Model file for the job. Use its own axes, mm. Round coordinates to 2 decimals unless told otherwise and drop trailing zeros. Use one line per item in the form item = value.
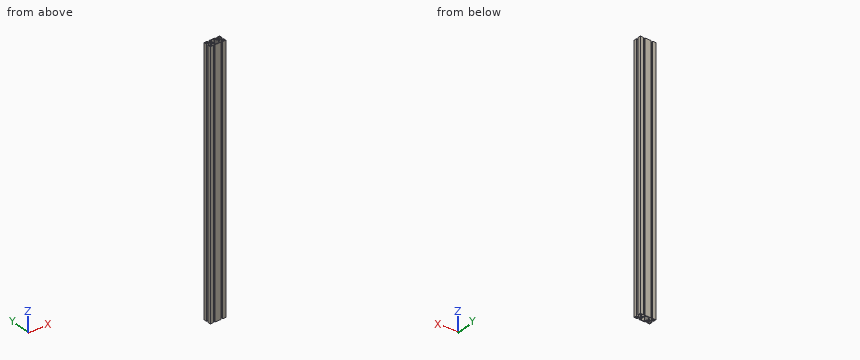
from build123d import *

# Parameters (mm, degrees)
F0_R     = 3
F0_R_2   = 2.5
F1_DEPTH = 1000
F2_R     = 2
F3_R     = 7


# Not quite as in the source:
# - a feature names something its author has since deleted; it is built from what else it names


with BuildPart() as f1:
    # F0 (on Top) → F1 (new body)
    with BuildSketch(Plane.XY):
        with BuildLine():
            Line((18.15, -15), (30, -15))
            Line((30, -15), (30, -3.15))
            Line((30, -3.15), (27.5, -3.15))
            Line((27.5, -3.15), (27.5, -5.15))
            Line((27.5, -5.15), (21.5477069044, -5.15))
            ThreePointArc((21.5477069044, -5.15), (19.5, 0), (21.5477069044, 5.15))
            Line((21.5477069044, 5.15), (27.5, 5.15))
            Line((27.5, 5.15), (27.5, 3.15))
            Line((27.5, 3.15), (30, 3.15))
            Line((30, 3.15), (30, 15))
            Line((30, 15), (18.15, 15))
            Line((18.15, 15), (18.15, 12.5))
            Line((18.15, 12.5), (20.15, 12.5))
            Line((20.15, 12.5), (20.15, 6.5477069044))
            ThreePointArc((20.15, 6.5477069044), (15, 4.5), (9.85, 6.5477069044))
            Line((9.85, 6.5477069044), (9.85, 12.5))
            Line((9.85, 12.5), (11.85, 12.5))
            Line((11.85, 12.5), (11.85, 15))
            Line((11.85, 15), (-11.85, 15))
            Line((-11.85, 15), (-11.85, 12.5))
            Line((-11.85, 12.5), (-9.85, 12.5))
            Line((-9.85, 12.5), (-9.85, 6.5477069044))
            ThreePointArc((-9.85, 6.5477069044), (-15, 4.5), (-20.15, 6.5477069044))
            Line((-20.15, 6.5477069044), (-20.15, 12.5))
            Line((-20.15, 12.5), (-18.15, 12.5))
            Line((-18.15, 12.5), (-18.15, 15))
            Line((-18.15, 15), (-30, 15))
            Line((-30, 15), (-30, 3.15))
            Line((-30, 3.15), (-27.5, 3.15))
            Line((-27.5, 3.15), (-27.5, 5.15))
            Line((-27.5, 5.15), (-21.5477069044, 5.15))
            ThreePointArc((-21.5477069044, 5.15), (-19.5, 0), (-21.5477069044, -5.15))
            Line((-21.5477069044, -5.15), (-27.5, -5.15))
            Line((-27.5, -5.15), (-27.5, -3.15))
            Line((-27.5, -3.15), (-30, -3.15))
            Line((-30, -3.15), (-30, -15))
            Line((-30, -15), (-18.15, -15))
            Line((-18.15, -15), (-18.15, -12.5))
            Line((-18.15, -12.5), (-20.15, -12.5))
            Line((-20.15, -12.5), (-20.15, -6.5477069044))
            ThreePointArc((-20.15, -6.5477069044), (-15, -4.5), (-9.85, -6.5477069044))
            Line((-9.85, -6.5477069044), (-9.85, -12.5))
            Line((-9.85, -12.5), (-11.85, -12.5))
            Line((-11.85, -12.5), (-11.85, -15))
            Line((-11.85, -15), (11.85, -15))
            Line((11.85, -15), (11.85, -12.5))
            Line((11.85, -12.5), (9.85, -12.5))
            Line((9.85, -12.5), (9.85, -6.5477069044))
            ThreePointArc((9.85, -6.5477069044), (15, -4.5), (20.15, -6.5477069044))
            Line((20.15, -6.5477069044), (20.15, -12.5))
            Line((20.15, -12.5), (18.15, -12.5))
            Line((18.15, -12.5), (18.15, -15))
        make_face()
        with Locations((-25, -10)):
            Circle(F0_R, mode=Mode.SUBTRACT)
        with Locations((25, -10)):
            Circle(F0_R, mode=Mode.SUBTRACT)
        with Locations((-15, 0)):
            Circle(F0_R_2, mode=Mode.SUBTRACT)
        with Locations((-25, 10)):
            Circle(F0_R, mode=Mode.SUBTRACT)
        Polygon((-7, 7), (-7, 12.5), (0, 12.5), (7, 12.5), (7, 7), (10, 0), (7, -7), (7, -12.5), (0, -12.5), (-7, -12.5), (-7, -7), (-10, 0), align=None, mode=Mode.SUBTRACT)
        with Locations((15, 0)):
            Circle(F0_R_2, mode=Mode.SUBTRACT)
        with Locations((25, 10)):
            Circle(F0_R, mode=Mode.SUBTRACT)
    extrude(amount=F1_DEPTH)

    # F2
    f2_edges = [f1.edges().sort_by_distance(p)[0] for p in [
        (-7, 12.5, 500),
        (7, 12.5, 500),
    ]]
    fillet(f2_edges, radius=F2_R)

    # F3
    f3_edges = [f1.edges().sort_by_distance(p)[0] for p in [
        (-7, 7, 500),
        (-10, 0, 500),
        (7, 7, 500),
        (10, 0, 500),
    ]]
    fillet(f3_edges, radius=F3_R)


solid = f1.part
1. Flat gauge pins, fed straight in: pin 1 (5.5 mm diameter, centred on x = 25, y = -10, fed in from +Z); pin 2 (8 mm diameter, centred on x = -15, y = 0, fed in from -Z). Where does each tip first touch, or does it go through?
Geometry check:
pin_1 = through
pin_2 = 0
2. Cut at A-A, the plane z = 240. Give the number of separate pieces and of enclosed holes in the cut face, plus the area to 3 significant figures.
Geometry check:
separate_pieces = 1
enclosed_holes = 7
area = 710 mm^2
3. Wall check: probe 1 along X at (y, z) = (-0.5, 414.5); probe 2 along X at (y, z) = (-11, 909.5); probe 3 along Y at (x, z) = (10, 126.5). Give the ranges that are in metal, low to high.
Geometry check:
probe_1 = -19.52 to -17.45, -12.55 to -9.37, 9.37 to 12.55, 17.45 to 19.52
probe_2 = -30 to -27.83, -22.17 to -20.15, -9.85 to -7, 7 to 9.85, 20.15 to 22.17, 27.83 to 30
probe_3 = -15 to -12.5, -6.41 to 6.41, 12.5 to 15
